from build123d import *

# Parameters (mm, degrees)
SKETCH1_W           = 6.5
SKETCH1_H           = 5.5
BOSS_EXTRUDE1_DEPTH = 184
CUT_EXTRUDE2_DEPTH  = 185
SKETCH3_W           = 1.5
SKETCH3_H           = 6.243718407
SKETCH3_H_2         = 7.062553001
BOSS_EXTRUDE2_DEPTH = 6
SKETCH4_R           = 1.4
CUT_EXTRUDE3_DEPTH  = 7.5
FILLET1_R           = 1
BOSS_EXTRUDE3_DEPTH = 6
BOSS_EXTRUDE4_DEPTH = 6


with BuildPart() as part:
    # Sketch1 → Boss-Extrude1 (new body)
    with BuildSketch(Plane.XY):
        with Locations((3.25, 2.75)):
            Rectangle(SKETCH1_W, SKETCH1_H)
    extrude(amount=BOSS_EXTRUDE1_DEPTH)

    # Sketch2 → Cut-Extrude2 (cut, through all)
    with BuildSketch(Plane(origin=(0, 0, 0), x_dir=(-1, 0, 0), z_dir=(0, 0, -1))):
        Polygon((0, 1), (-6.5, 5.5), (0, 5.5), align=None)
    extrude(amount=-CUT_EXTRUDE2_DEPTH, mode=Mode.SUBTRACT)

    # Sketch3 → Boss-Extrude2 (add)
    with BuildSketch(Plane.XZ):
        with Locations((0.75, 3.121859204)):
            Rectangle(SKETCH3_W, SKETCH3_H)
        with Locations((0.75, 180.4687235)):
            Rectangle(SKETCH3_W, SKETCH3_H_2)
    extrude(amount=BOSS_EXTRUDE2_DEPTH)

    # Sketch4 → Cut-Extrude3 (cut, through all)
    with BuildSketch(Plane.ZY):
        with Locations((180.937446999, -3)):
            Circle(SKETCH4_R)
    cut_extrude3 = extrude(amount=-CUT_EXTRUDE3_DEPTH, mode=Mode.SUBTRACT)

    # Mirror1: Cut-Extrude3 across plane
    add(cut_extrude3.mirror(Plane.XY.offset(92)), mode=Mode.SUBTRACT)

    # Fillet1
    fillet1_edges = [part.edges().sort_by_distance(p)[0] for p in [
        (0.75, -6, 6.243718407),
        (0.75, -6, 0),
        (0.75, -6, 184),
        (0.75, -6, 176.937446999),
    ]]
    fillet(fillet1_edges, radius=FILLET1_R)

    # Sketch5 → Boss-Extrude3 (add)
    with BuildSketch(Plane(origin=(0, 0, 0), x_dir=(-1, 0, 0), z_dir=(0, 0, -1))):
        Polygon((-6.5, 0), (-6.5, 5.5), (-1.5, 2.038461538), (-1.5, 0), align=None)
    extrude(amount=BOSS_EXTRUDE3_DEPTH)

    # Sketch6 → Boss-Extrude4 (add)
    with BuildSketch(Plane.XY.offset(184)):
        Polygon((6.5, 5.5), (6.5, 0), (1.5, 0), (1.5, 2.038461538), align=None)
    extrude(amount=BOSS_EXTRUDE4_DEPTH)


solid = part.part
For this review, take the finished solid that the model builds, in its own axes (mm). A direction names the side the tool comes from. Round coordinates to 2 decimals unless told otherwise and drop trailing zeros. Loops run counter-clockwise (first coordinate to the right, second up) from the corner with the lowest first, then second, coordinate; pieces in that order, holes last. Notation, with made-up numbers: (-27.75, 51.5) - (-11.75, 51.5) arc R29 cw to (-11.75, 76.5) - close; hole circle Ø11 at (53, 79). An arc over 180 degrees is marked (long way). One line per item, written item: value. Start each with the question number.
Item 1: The part is to be moulded in two halves that separate along Z. For faces 1 (the flat face through (3, 0, 91)), 2 (the flat face through (5, 2, 190)), 3 (the flat face through (5, 2, -6)), 4 (the flat face through (1.5, -1.6, 179.6)), say which applies: +Z half, -Z half, draft (parallel to the pull), parting line (faces both ways), or undercut.
Item 2: For faces 5 (the flat face through (1.5, -1.6, 3.8)), 6 (the flat face through (6.5, 3, 91)), list the 3-axis set-ups (+Z, -Z, +X, -X, +Y, -Y) from which the entire face can be reached by the end or side of a thin tool; tool diameter is ignored.
Item 3: Clearance check with flat-ended pins moving along their axes: pin 1 Ø1.5 at (x, y) = (1, -3.5) entering from +Z; pin 2 Ø1.2 at (x, y) = (1, -1.5) entering from -Z; pin 3 Ø1.6 at (y, z) = (1.5, 186) entering from -X; pin 4 Ø3 at (x, y) = (1, -0.5) entering from -Z. State where each tip first meets the part, or that it passes through.
Item 4: For L1, parallel to X at y = -0.25, z = 180; L2, parallel to Y at x = 1, z = 169; L3, parallel to Y at x = 4.5, z = 36.5, list the stretches that pass through material, from the lowest coordinate up.
Item 5: Take a section at A-A (z = 65). Give the boundary of the cut face in (x, y).
Answer below:
1. face 1: undercut
1. face 2: +Z half
1. face 3: -Z half
1. face 4: draft
2. face 5: +Z, -Z, +X, -Y
2. face 6: +Z, -Z, +X, +Y, -Y
3. pin 1: stops at z = 184
3. pin 2: stops at z = 0
3. pin 3: stops at x = 1.5
3. pin 4: stops at z = -6
4. L1: x = 0 to 1.5
4. L2: y = 0 to 1.69
4. L3: y = 0 to 4.12
5. outline: (0, 0) - (6.5, 0) - (6.5, 5.5) - (0, 1) - close
